```python
from build123d import *

# Parameters (mm, degrees)
F1_DEPTH      = 10.5
F2_W          = 140
F2_H          = 75
F3_DEPTH      = 5
F5_DEPTH      = 37.5
F5_DEPTH_BACK = 37.5
F6_DEPTH      = 10.5
F7_W          = 5
F7_H          = 75
F8_DEPTH      = 13.33


with BuildPart() as f1:
    # F0 (on Top) → F1 (new body)
    with BuildSketch(Plane.XY):
        with BuildLine():
            Line((-70, -37.5), (70, -37.5))
            Line((70, -37.5), (70, -5.5))
            Line((70, -5.5), (34.311988, -5.5))
            ThreePointArc((34.311988, -5.5), (-34.75, 0), (34.311988, 5.5))
            Line((34.311988, 5.5), (70, 5.5))
            Line((70, 5.5), (70, 37.5))
            Line((70, 37.5), (-70, 37.5))
            Line((-70, 37.5), (-70, -37.5))
        make_face()
    extrude(amount=F1_DEPTH)

    # F2 (on Top) → F3 (join)
    with BuildSketch(Plane.XY):
        Rectangle(F2_W, F2_H)
    extrude(amount=-F3_DEPTH)

    # F4 (on Front) → F5 (join, two sides)
    with BuildSketch(Plane.XZ) as f5_sk:
        Polygon((70, 10.5), (-70, 10.5), (-70, -5), (-65.432164, -2.96656), (-64.526948, -5), (70, -5), align=None)
        Polygon((-70, -5), (-70, 10.5), (-75.75882, 7.936376), align=None)
        Polygon((-64.526948, -5), (-70, -5), (-46.844684, -57.015147), (-42.276849, -54.981707), align=None)
    extrude(amount=F5_DEPTH)
    extrude(f5_sk.sketch, amount=-F5_DEPTH_BACK)

    # F0 (on Top) → F6 (cut, through all)
    with BuildSketch(Plane.XY):
        with BuildLine():
            Line((34.311988, -5.5), (70, -5.5))
            Line((70, -5.5), (70, 5.5))
            Line((70, 5.5), (34.311988, 5.5))
            ThreePointArc((34.311988, 5.5), (-34.75, 0), (34.311988, -5.5))
        make_face()
    extrude(amount=F6_DEPTH, mode=Mode.SUBTRACT)

    # F7 (on face) → F8 (join)
    with BuildSketch(Plane.XY.offset(10.5)):
        with Locations((-67.5, 0)):
            Rectangle(F7_W, F7_H)
    extrude(amount=F8_DEPTH)


solid = f1.part
```
Here's how the part is built. I have some questions about the finished solid (model axes, mm). A direction names the side the tool comes from. Round coordinates to 2 decimals unless told otherwise and drop trailing zeros. Loops run counter-clockwise (first coordinate to the right, second up) from the corner with the lowest first, then second, coordinate; pieces in that order, holes last. Notation, with made-up numbers: (50.5, 48.25) -> (65.5, 48.25) arc R26 cw to (65.5, 72.25) -> close; hole circle Ø1 at (-14.75, -38.75). An arc over 180 degrees is marked (long way). Answer as CSV lines item,"result". Start each with the question number.
1. Imagine slicing it at A-A on x = 0. Write out the boundary of the cut face in (y, z).
2. If we mould it in two halves opening along Y, with no side actions, what happens to faces 1 (the face through (52, 5.5, 5)), 2 (the face through (2, 1, -5)), 3 (the face through (-9, 37.5, 1))? For each: pulls with the +Y half, pulls with the -Y half, needs draft (parallel to the pull), parting line crosses it, or undercut.
3. Imagine slicing it at D-D on z = 5. Write out the boundary of the cut face in (x, y).
4. Imagine slicing it at B-B on x = -49. Write out the boundary of the cut face in (y, z).
5. I'm going to push flat-ended pins straight in: P1, Ø14.5, axis at y = 4, z = 18.5, coming from the +X side; P2, Ø12, axis at x = 47.5, y = -2, coming from the +Z side; P3, Ø1.5, axis at y = -11, z = 7, coming from the -X side. Where does each tip first touch, or does it pass through?
6. I need wall thicknesses on probe 1 along Z at (x, y) = (-3, -2); probe 2 along Y at (x, z) = (0, 4); probe 3 along Z at (x, y) = (-37, 11). Which ranges of each line are inside material? Lowest first, please. Write a range as from..to.
7. For faces 4 (the face through (-70, -1, 17)), 5 (the face through (52, -5.5, 5)), 6 (the face through (-53.246, 0.525, -30.341)), 7 (the face through (5, 0, 0)), 8 (the face through (-65, -1, 17)), which set-ups out of +Z, -Z, +X, -X, +Y, -Y let a thin tool reach every point of the face, with its end or its side?
8. Imagine slicing it at C-C on y = 0. Write out the boundary of the cut face in (x, z), plus the area to 3 significant figures.
Solution:
1,outline,"(-37.5, -5) -> (37.5, -5) -> (37.5, 10.5) -> (34.75, 10.5) -> (34.75, 0) -> (-34.75, 0) -> (-34.75, 10.5) -> (-37.5, 10.5) -> close"
2,face 1,"undercut"
2,face 2,"needs draft"
2,face 3,"pulls with the +Y half"
3,outline,"(-74.45, -37.5) -> (70, -37.5) -> (70, -5.5) -> (34.31, -5.5) arc R34.75 cw (long way) to (34.31, 5.5) -> (70, 5.5) -> (70, 37.5) -> (-74.45, 37.5) -> close"
4,outline,"(-37.5, -52.17) -> (37.5, -52.17) -> (37.5, -39.88) -> (-37.5, -39.88) -> close; (-37.5, -5) -> (37.5, -5) -> (37.5, 10.5) -> (-37.5, 10.5) -> close"
5,P1,"x = -65"
5,P2,"z = 10.5"
5,P3,"x = -75.68"
6,probe 1,"-5..0"
6,probe 2,"-37.5..-34.75, 34.75..37.5"
6,probe 3,"-5..10.5"
7,face 4,"+Z, -X, +Y, -Y"
7,face 5,"+Z, +X"
7,face 6,"+X, +Y, -Y"
7,face 7,"+Z"
7,face 8,"+Z, +X, +Y, -Y"
8,outline,"(-75.76, 7.94) -> (-46.84, -57.02) -> (-42.28, -54.98) -> (-64.53, -5) -> (70, -5) -> (70, 0) -> (-34.75, 0) -> (-34.75, 10.5) -> (-65, 10.5) -> (-65, 23.83) -> (-70, 23.83) -> (-70, 10.5) -> close"
8,area,"1,460 mm²"
